from build123d import *

# Parameters (mm, degrees)
F1_DEPTH    = 130
F2_R        = 2
F3_T1_DEPTH = 130
F3_T4_ANGLE = 148.4890190499
F3_T6_ANGLE = 148.4890190499
F4_W        = 18
F4_H        = 116
F5_DEPTH    = 15
F6_W        = 100
F6_H        = 140.9174852884
F6_H_2      = 11.4719050156
F1_FACE2_W  = 126
F1_FACE2_H  = 170.8886996293
F7_DEPTH    = 300
F8_R        = 2


# Not quite as in the source:
# - a fillet or chamfer that OpenCascade refuses, or shapes differently, is made with other operations: its cross-section is extruded or revolved along the edge and cut away or added


with BuildPart() as f1:
    # F0 (on Front) → F1 (new body)
    with BuildSketch(Plane.XZ):
        Polygon((-46.5874281185, -17.2704798563), (-66.5874281185, -17.2704798563), (-62.7051424419, -2.781592462), (-71.2205818073, -4.9188610433), (-76.3969627094, -24.2373775691), (-40.1931625425, -24.2373775691), (0, 125.7655471563), (44.4641634577, -24.2373775691), (53.6030372906, -24.2373775691), (0, 156.5961688757), align=None)
    extrude(amount=F1_DEPTH)

    # F2
    f2_edges = [f1.edges().sort_by_distance(p)[0] for p in [
        (-23.293714, -130, 69.662845),
        (-20.096581, -130, 50.764085),
        (-64.646285, -130, -10.026036),
        (-62.705142, -65, -2.781592),
        (-71.220582, -65, -4.918861),
        (22.232082, -130, 50.764085),
        (26.801519, -130, 66.179396),
        (-23.293714, 0, 69.662845),
        (-20.096581, 0, 50.764085),
        (-56.587428, 0, -17.27048),
        (-64.646285, 0, -10.026036),
        (-66.962862, 0, -3.850227),
        (-73.808772, 0, -14.578119),
        (-58.295063, 0, -24.237378),
        (22.232082, 0, 50.764085),
        (49.0336, 0, -24.237378),
        (26.801519, 0, 66.179396),
        (-58.295063, -130, -24.237378),
        (49.0336, -130, -24.237378),
    ]]
    fillet(f2_edges, radius=F2_R)

    # F3: fillet of radius 5 on 1 edges, made by hand

    # F3_s2 → F3_t1 (cut)
    with BuildSketch(Plane.XZ):
        with BuildLine():
            ThreePointArc((-4.5868330474, 139.4778748971), (0.1768690132, 143.1833450148), (5.0366225074, 139.6047751759))
            Line((5.0366225074, 139.6047751759), (0, 156.5961688757))
            Line((0, 156.5961688757), (-4.5868330474, 139.4778748971))
        make_face()
    extrude(amount=F3_T1_DEPTH, mode=Mode.SUBTRACT)

    # F3_s3 → F3_t4 (revolve, cut)
    with BuildSketch(Plane(origin=(34.5622091716, 0, 128.9879206501), x_dir=(0, 1, 0), z_dir=(-0.2588190451, 0, -0.9659258263))):
        with BuildLine():
            ThreePointArc((0, -38.5300708951), (-0.5857864376, -39.9442844575), (-2, -40.5300708951))
            Line((-2, -40.5300708951), (0, -40.5300708951))
            Line((0, -40.5300708951), (0, -38.5300708951))
        make_face()
    revolve(axis=Axis((0.2427960841, 0, 138.1837796716), (0, 1, 0)), revolution_arc=F3_T4_ANGLE, mode=Mode.SUBTRACT)

    # F3_s5 → F3_t6 (revolve, cut)
    with BuildSketch(Plane(origin=(-37.6327378938, 0, 126.9566390213), x_dir=(0, 1, 0), z_dir=(0.2841991009, 0, -0.9587652847))):
        with BuildLine():
            ThreePointArc((-130, 42.5044903939), (-129.4142135624, 43.9187039563), (-128, 44.5044903939))
            Line((-128, 44.5044903939), (-130, 44.5044903939))
            Line((-130, 44.5044903939), (-130, 42.5044903939))
        make_face()
    revolve(axis=Axis((0.2427960841, -130, 138.1837796716), (0, -1, 0)), revolution_arc=F3_T6_ANGLE, mode=Mode.SUBTRACT)

    # F4 (on face) → F5 (cut)
    with BuildSketch(Plane(origin=(0, 0, -24.2373775691), x_dir=(1, 0, 0), z_dir=(0, 0, -1))):
        with Locations((-54.3969627094, 65)):
            Rectangle(F4_W, F4_H)
    extrude(amount=-F5_DEPTH, mode=Mode.SUBTRACT)

    # F6 (on face) + F1_face2 (on face) → F7 (cut)
    with BuildSketch(Plane(origin=(-39.1490422189, 0, 10.489954247), x_dir=(0, -1, 0), z_dir=(-0.9659258263, 0, 0.2588190451))):
        with Locations((65, 63.0793791654)):
            Rectangle(F6_W, F6_H)
        with Locations((65, 139.2740743175)):
            Rectangle(F6_W, F6_H_2)
    with BuildSketch(Plane(origin=(29.319829899, -65, 57.6836988034), x_dir=(0, 1, 0), z_dir=(0.9587652847, 0, 0.2841991009))):
        Rectangle(F1_FACE2_W, F1_FACE2_H)
    extrude(amount=-F7_DEPTH, dir=(-0.9659258263, 0, 0.2588190451), mode=Mode.SUBTRACT)

    # F8
    f8_edges = [f1.edges().sort_by_distance(p)[0] for p in [
        (-22.822898, -15, 71.419956),
        (28.960029, -115, 58.897511),
        (-22.822898, -115, 71.419956),
        (0.176869, -115, 143.183345),
        (28.960029, -15, 58.897511),
        (0.176869, -15, 143.183345),
    ]]
    fillet(f8_edges, radius=F8_R)


solid = f1.part
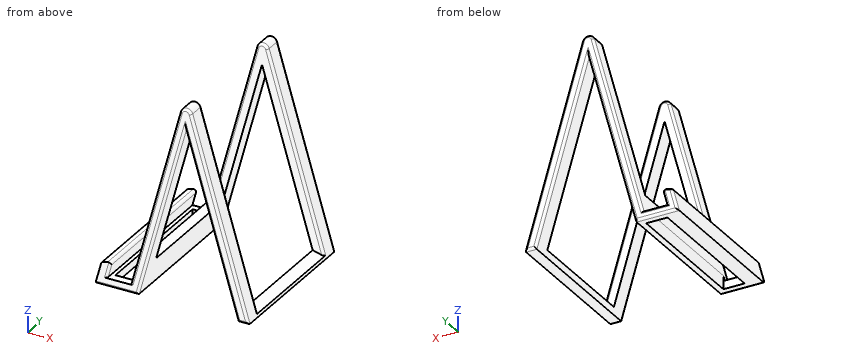
Build history of the part. All positions in model axes, mm. Coordinates: 2 decimals unless noted, no trailing zeros. Order: outer loops, then holes, each group sorted by start corner. A loop starts at its lowest first (then second) coordinate and runs counter-clockwise, first axis right, second up. Notation, with made-up numbers: M 76,69.25 L 104,69.25 A21 cw 104,81.25 Z; hole C 67.25,69.5 d5. An arc over 180 degrees is marked long. One line per question, with ' | ' between items. Start each with the question number.
Q1. Probe L1, parallel to X at y = -13, z = 123.5; L2, parallel to Y at x = -11.5, z = 89.5; L3, parallel to Y at x = 35, z = 37. List the from-to ranges inside material, lowest first. Write a range as from..to.
Q2. Saw through at C-C (z = 40). Count the separate pieces of the cut face and the enclosed holes in it, then the cut area to 3 significant figures.
Q3. Saw through at A-A (y = -74). List the corners of the cut face in (x, z), then the cut area to 3 significant figures.
Q4. Flat gauge pins, fed straight in: pin 1 Ø9 at (y, z) = (-77, -19.5) entering from -X; pin 2 Ø12.5 at (x, z) = (-57, -16.5) entering from -Y. Where does each tip first touch, or does it go through?
Q5. Saw through at B-B (x = -54). List the corners of the cut face in (y, z).
Check values:
1) L1: x = -8.87..-0.61, 0.67..9.81 | L2: y = -129.98..-115, -15..-0.02 | L3: y = -129.24..-115.76, -14.24..-0.76
2) separate pieces: 4 | enclosed holes: 0 | area: 511 mm2
3) outline: M -76.4,-24.24 L -63.4,-24.24 L -63.4,-17.27 L -66.59,-17.27 L -63.59,-6.07 A2 ccw -66,-3.61 L -70.08,-4.63 A2 ccw -71.52,-6.05 Z; M -45.4,-24.24 L -40.19,-24.24 L -33.35,1.3 L -41.06,3.36 L -45.4,-12.83 Z; M 42.96,-19.15 L 44.46,-24.24 L 53.6,-24.24 L 52.88,-21.81 Z | area: 424 mm2
4) pin 1: stops at x = -76.33 | pin 2: stops at y = -130
5) outline: M -130,-22.24 A2 ccw -128,-24.24 L -123,-24.24 L -123,-17.27 L -130,-17.27 Z; M -7,-24.24 L -2,-24.24 A2 ccw 0,-22.24 L 0,-19.27 A2 ccw -2,-17.27 L -7,-17.27 Z
